Autodesk Inventor part; units mm, degrees
ref_plane "YZ Plane" through (0, 0, 0) normal (1, 0, 0) x (0, 1, 0)
ref_plane "XZ Plane" through (0, 0, 0) normal (0, 1, 0) x (-1, 0, 0)
ref_plane "XY Plane" through (0, 0, 0) normal (0, 0, 1) x (1, 0, 0)
sketch "Szkic1" plane through (0, 0, 0) normal (0, 1, 0) x (-1, 0, 0)
  line L0 (-22.55, -41.4) -> (22.55, -41.4)
  line L1 (22.55, -41.4) -> (22.55, 41.4)
  line L2 (22.55, 41.4) -> (-22.55, 41.4)
  line L3 (-22.55, 41.4) -> (-22.55, -41.4)
  line L4 (-22.55, -41.4) -> (22.55, 41.4) construction
  line L5 (22.55, -41.4) -> (-22.55, 41.4) construction
  point P0 (0, 0)
  dimension "d0" = 45.1
  dimension "d1" = 82.8
extrude "Wyciągnięcie proste1" add sketch "Szkic1" along normal blind 3
sketch "Szkic2" plane through (0, 3, 0) normal (0, 1, 0) x (1, 0, 0)
  line L0 (22.55, 41.4) -> (-22.55, 41.4)
  line L1 (-22.55, 41.4) -> (-22.55, -41.4)
  line L2 (-22.55, -41.4) -> (22.55, -41.4)
  line L3 (22.55, -41.4) -> (22.55, 41.4)
  point P0 (0, 0)
  point P1 (-16.95, -16.1)
  point P2 (19.05, 37.9)
  dimension "d4" = 57.5
  dimension "d5" = 54
  dimension "d6" = 3.5
  dimension "d7" = 36
hole "Otwór1" at (-16.95, 3, 16.1) at (19.05, 3, -37.9) direction (0, -1, 0) diameter 3.5 end through all
sketch "Szkic3" plane through (0, 3, 0) normal (0, 1, 0) x (1, 0, 0)
  circle A0 centre (-16.95, -16.1) radius 1.75
  circle A1 centre (19.05, 37.9) radius 1.75
  line L0 (22.55, 41.4) -> (-22.55, 41.4)
  line L1 (-22.55, 41.4) -> (-22.55, -41.4)
  line L2 (-22.55, -41.4) -> (22.55, -41.4)
  line L3 (22.55, -41.4) -> (22.55, 41.4)
  line L4 (-21.55, -40.9) -> (-1.05, -40.9)
  line L5 (-1.05, -40.9) -> (-1.05, -31.9)
  line L6 (-1.05, -31.9) -> (-21.55, -31.9)
  line L7 (-21.55, -31.9) -> (-21.55, -40.9)
  line L8 (0.95, -40.9) -> (21.45, -40.9)
  line L9 (21.45, -40.9) -> (21.45, -31.9)
  line L10 (21.45, -31.9) -> (0.95, -31.9)
  line L11 (0.95, -31.9) -> (0.95, -40.9)
  line L12 (0.95, -30.9) -> (21.45, -30.9)
  line L13 (21.45, -30.9) -> (21.45, -21.9)
  line L14 (21.45, -21.9) -> (0.95, -21.9)
  line L15 (0.95, -21.9) -> (0.95, -30.9)
  line L16 (20.55, 34.7531) -> (11.55, 34.7531)
  line L17 (11.55, 34.7531) -> (11.55, 14.2531)
  line L18 (11.55, 14.2531) -> (20.55, 14.2531)
  line L19 (20.55, 14.2531) -> (20.55, 34.7531)
  line L20 (10.4919, 34.7531) -> (1.4919, 34.7531)
  line L21 (1.4919, 34.7531) -> (1.4919, 14.2531)
  line L22 (1.4919, 14.2531) -> (10.4919, 14.2531)
  line L23 (10.4919, 14.2531) -> (10.4919, 34.7531)
  line L24 (21.45, 12.0004) -> (12.45, 12.0004)
  line L25 (12.45, 12.0004) -> (12.45, -17.9996)
  line L26 (12.45, -17.9996) -> (21.45, -17.9996)
  line L27 (21.45, -17.9996) -> (21.45, 12.0004)
  line L28 (-20.8756, 23.1013) -> (-11.8756, 23.1013)
  line L29 (-11.8756, 23.1013) -> (-11.8756, 2.6013)
  line L30 (-11.8756, 2.6013) -> (-20.8756, 2.6013)
  line L31 (-20.8756, 2.6013) -> (-20.8756, 23.1013)
  point P0 (0, 0)
  dimension "d15" = 20.5
  dimension "d16" = 9
  dimension "d17" = 1
  dimension "d18" = 0.5
  dimension "d19" = 20.5
  dimension "d20" = 9
  dimension "d21" = 2
  dimension "d22" = 0.5
  dimension "d23" = 20.5
  dimension "d24" = 9
  dimension "d25" = 1
  dimension "d26" = 9
  dimension "d27" = 20.5
  dimension "d28" = 9
  dimension "d29" = 20.5
  dimension "d30" = 9
  dimension "d31" = 30
  dimension "d32" = 9
  dimension "d33" = 20.5
extrude "Wyciągnięcie proste2" add sketch "Szkic3" along normal blind 8 contours L7 L6 L5 L4 | L11 L10 L9 L8 | L15 L14 L13 L12 | L19 L18 L17 L16 | L23 L22 L21 L20 | L27 L26 L25 L24 | L28 L29 L30 L31
properties part number "RBC4242"
Can you work these out from the model? Positions are in its coordinate system, mm. A direction names the side the tool comes from. Coordinates: 2 decimals unless noted, no trailing zeros. Loops run counter-clockwise (first coordinate to the right, second up) from the corner with the lowest first, then second, coordinate; pieces in that order, holes last. Notation, with made-up numbers: (50, 19) - (102, 19) arc R20 ccw to (102, 45) - close; hole circle Ø6 at (-39.75, 66.25). An arc over 180 degrees is marked (long way). Answer as CSV lines item,"result". Start each with the question number.
1) Suppose I cut it at A-A (x = 19.05). Please give me the cut outline in (y, z), plus the area to 3 significant figures.
2) Thinking about a two-plate mould opening in Z: for faces 4 (the flat face through (21.45, 7, 26)), 5 (the flat face through (-16, 7, -23.101)), 6 (the flat face through (16, 7, -14.253)), which applies, pulls with the +Z half, pulls with the -Z half, needs draft (parallel to the pull), parting line crosses it, or undercut?
3) Suppose I cut it at B-B (z = 16.1). Please give me the cut outline in (x, y).
4) Suppose I cut it at C-C (y = 7). Please give me the cut outline in (x, z), plus the area to 3 significant figures.
5) Which directions (+Z, -Z, +X, -X, +Y, -Y) give clear straight access to the entire face, cutting with the end or side of a thin tool? Please do faces 1 (the flat face through (0.95, 7, 26)), 2 (the flat face through (21.45, 7, 3)), 3 (the flat face through (1.492, 7, -25)).
6) I need wall thicknesses on line 1 (Z direction, x = 19.5, y = 3.25); line 2 (X direction, y = 2.15, z = 16.1); line 3 (X direction, y = 7, z = 36). Which ranges of each line are inside material? Lowest first, please. Write a range as from..to.
7) Suppose I cut it at D-D (x = 14.5). Please give me the cut outline in (y, z), plus the area to 3 significant figures.
8) For pin 1 (4 mm diameter, centred on y = 9, z = 37.5, fed in from +X); pin 2 (4 mm diameter, centred on x = 5, y = 8, fed in from +Z); pin 3 (6.5 mm diameter, centred on y = 7, z = -20, fed in from +X), each with a flat end and sliding along its axis, tell me the tip position at first contact or that it passes through.
Check result:
1,outline,"(0, -41.4) - (3, -41.4) - (3, -39.65) - (0, -39.65) - close; (0, -36.15) - (3, -36.15) - (3, -34.75) - (11, -34.75) - (11, -14.25) - (3, -14.25) - (3, -12) - (11, -12) - (11, 18) - (3, 18) - (3, 21.9) - (11, 21.9) - (11, 30.9) - (3, 30.9) - (3, 31.9) - (11, 31.9) - (11, 40.9) - (3, 40.9) - (3, 41.4) - (0, 41.4) - close"
1,area,"786 mm²"
2,face 4,"needs draft"
2,face 5,"pulls with the -Z half"
2,face 6,"undercut"
3,outline,"(-22.55, 0) - (-18.7, 0) - (-18.7, 3) - (-22.55, 3) - close; (-15.2, 0) - (22.55, 0) - (22.55, 3) - (21.45, 3) - (21.45, 11) - (12.45, 11) - (12.45, 3) - (-15.2, 3) - close"
4,outline,"(-21.55, 31.9) - (-1.05, 31.9) - (-1.05, 40.9) - (-21.55, 40.9) - close; (-20.88, -23.1) - (-11.88, -23.1) - (-11.88, -2.6) - (-20.88, -2.6) - close; (0.95, 21.9) - (21.45, 21.9) - (21.45, 30.9) - (0.95, 30.9) - close; (0.95, 31.9) - (21.45, 31.9) - (21.45, 40.9) - (0.95, 40.9) - close; (1.49, -34.75) - (10.49, -34.75) - (10.49, -14.25) - (1.49, -14.25) - close; (11.55, -34.75) - (20.55, -34.75) - (20.55, -14.25) - (11.55, -14.25) - close; (12.45, -12) - (21.45, -12) - (21.45, 18) - (12.45, 18) - close"
4,area,"1,380 mm²"
5,face 1,"+Z, -Z, -X, +Y"
5,face 2,"+Z, -Z, +X, +Y"
5,face 3,"-Z, +Y"
6,line 1,"z = -34.75..-14.25, -12..18, 21.9..30.9, 31.9..40.9"
6,line 2,"x = -22.55..-18.7, -15.2..22.55"
6,line 3,"x = -21.55..-1.05, 0.95..21.45"
7,outline,"(0, -41.4) - (3, -41.4) - (3, -34.75) - (11, -34.75) - (11, -14.25) - (3, -14.25) - (3, -12) - (11, -12) - (11, 18) - (3, 18) - (3, 21.9) - (11, 21.9) - (11, 30.9) - (3, 30.9) - (3, 31.9) - (11, 31.9) - (11, 40.9) - (3, 40.9) - (3, 41.4) - (0, 41.4) - close"
7,area,"796 mm²"
8,pin 1,"stops at x = 21.45"
8,pin 2,"stops at z = 40.9"
8,pin 3,"stops at x = 20.55"
